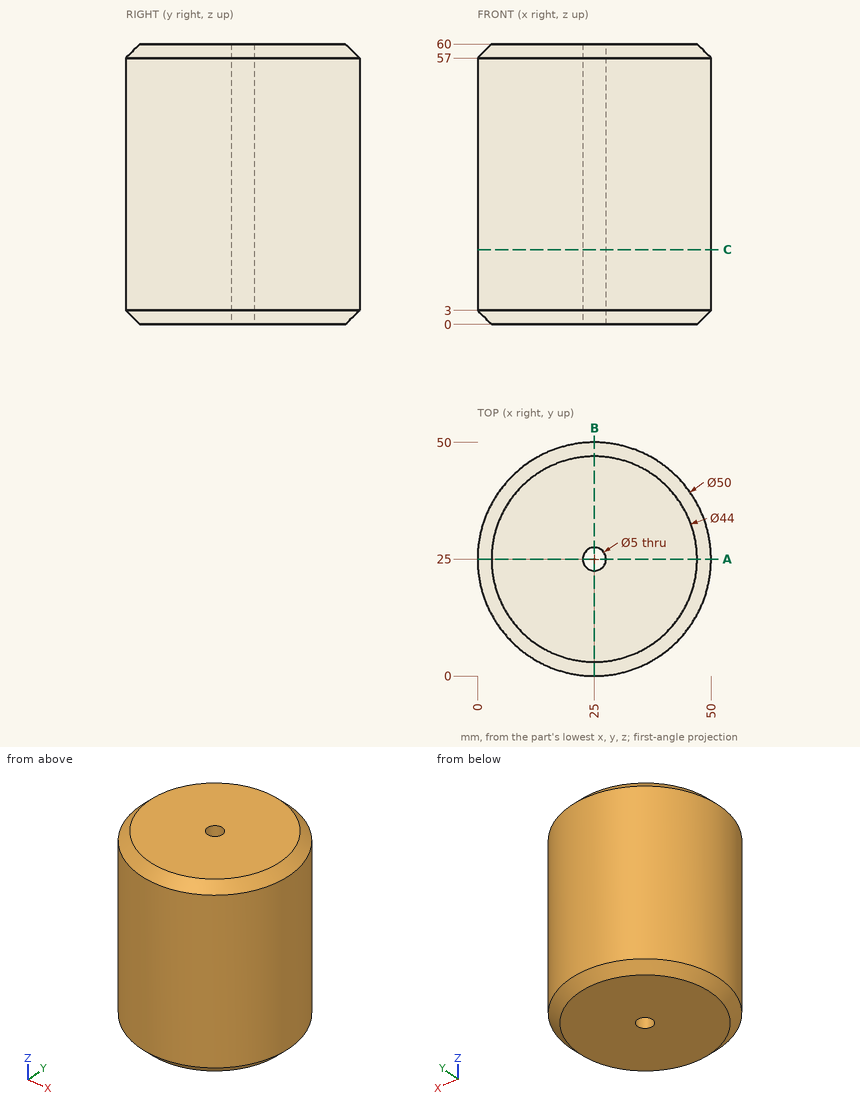
Geometry check sheet. Reference: drawing and pictorial views, mm from the part's lowest x, y, z. Give positions to 0.01 mm unless a question says otherwise; leave off trailing zeros. Write each loop counter-clockwise with the first axis right and the second up, starting at its lowest first coordinate (ties: lowest second). Pieces come first, ordered by that corner, then holes. Notation, with made-up numbers: M 35,65.5 L 87,65.5 A20 ccw 87,71.5 Z; hole C -14.5,62 d9. An arc over 180 degrees is marked long. Put each result on its own line as item: value. Start each with the question number.
1. Section check A-A (y = 25). Record the cut outline in (x, z), and give its area (3 significant figures).
2. Scan lines: line 1 along Y through (x, z) = (25, 16.5); line 2 along Y through (x, z) = (26, 23); line 3 along Y through (x, z) = (20, 23). Record each from-to range of solid material in increasing order. Write a range as [from, to].
3. Section check C-C (z = 16). Record the cut outline in (x, y).
4. Go/stop test with flat-tipped pins: pin 1 Ø8 at (x, z) = (23, 39) entering from +Y; pin 2 Ø1 at (x, z) = (32.5, 43.5) entering from -Y; pin 3 Ø4 at (x, z) = (33, 25.5) entering from -Y. Record where each tip stops, or that it passes through.
Answer list:
1. outline: M 0,3 L 3,0 L 22.5,0 L 22.5,60 L 3,60 L 0,57 Z; M 27.5,0 L 47,0 L 50,3 L 50,57 L 47,60 L 27.5,60 Z
1. area: 2,680 mm2
2. line 1: [0, 22.5], [27.5, 50]
2. line 2: [0.02, 22.71], [27.29, 49.98]
2. line 3: [0.51, 49.49]
3. outline: C 25,25 d50; hole C 25,25 d5
4. pin 1: y = 50
4. pin 2: y = 1
4. pin 3: y = 0.73
